Input: part model. Units: mm. Frame: model coordinates. Coordinates: 2 decimals unless noted, no trailing zeros. Loops run counter-clockwise (first coordinate to the right, second up) from the corner with the lowest first, then second, coordinate; pieces in that order, holes last. Notation, with made-up numbers: M 58.25,1.25 L 79.25,1.25 A25 cw 79.25,24.25 Z; hole C 38.5,-36.5 d9. An arc over 180 degrees is marked long. Use a Markdown table: item, result. Add a question column.
1. Section C-C on y = -47. Output: boundary loops of the cut face in (x, z), then the cut area to 3 significant figures.
2. Draft query along X for faces 1 (the flat face through (52, -17, 15)), 2 (the flat face through (54, -35, 15)), 3 (the cylindrical face through (38.49, -40.61, 14.93)). Return one class per face: +X half, -X half, draft (parallel to the pull), parting line (faces both ways), or undercut.
3. Section D-D on x = 19. Output: boundary loops of the cut face in (y, z).
4. Section B-B on z = 14.5. Output: boundary loops of the cut face in (x, y).
5. Section A-A on y = -21. Output: boundary loops of the cut face in (x, z), then the cut area to 3 significant figures.
6. Line query: L1, parallel to X at y = -34, z = 12.75; L2, parallel to X at y = -22, z = 13.25; L3, parallel to Y at x = -23.5, z = 15.5. Output: solid intervals per line, ascending. Write a range as [from, to].
7. Pin query (flat end, axial travel): pin 1 (6 mm diameter, centred on x = -21, z = 11, fed in from +Y); pin 2 (1.8 mm diameter, centred on x = 39.6, y = -39.6, fed in from -Z); pin 3 (2 mm diameter, centred on x = -31, z = 12, fed in from +Y). Return the tip coordinate at first contact, or that it passes through.
```python
from build123d import *

# Parameters (mm, degrees)
CYLINDER875_R               = 1.5
CYLINDER875_DEPTH           = 20
CYLINDER875_PLACEMENT_ANGLE = 45
CYLINDER866_R               = 1.5
CYLINDER866_DEPTH           = 20
CYLINDER869_R               = 1.5
CYLINDER869_DEPTH           = 20
CYLINDER869_PLACEMENT_ANGLE = 135
CYLINDER372_R               = 1.5
CYLINDER372_DEPTH           = 20
CYLINDER377_R               = 1.5
CYLINDER377_DEPTH           = 20
CYLINDER377_PLACEMENT_ANGLE = 225
CYLINDER876_R               = 1.5
CYLINDER876_DEPTH           = 20
CYLINDER873_R               = 1.5
CYLINDER873_DEPTH           = 20
CYLINDER873_PLACEMENT_ANGLE = 45
CYLINDER874_R               = 1.5
CYLINDER874_DEPTH           = 20
CYLINDER867_R               = 52
CYLINDER867_DEPTH           = 10
BOX134_W                    = 108
BOX134_H                    = 36
BOX134_DEPTH                = 10


with BuildPart() as obj1:
    # Cylinder875 → Cylinder875 (new body)
    with BuildSketch(Plane.XY):
        Circle(CYLINDER875_R)
    extrude(amount=CYLINDER875_DEPTH)


with BuildPart() as obj1_1:
    # Cylinder875 placement: moved
    add(obj1.part.moved(Location((39.59798, -39.59798, 2))).rotate(Axis((39.59798, -39.59798, 2), (0, 0, 1)), CYLINDER875_PLACEMENT_ANGLE))


with BuildPart() as obj2:
    # Cylinder866 → Cylinder866 (new body)
    with BuildSketch(Plane(origin=(56, 0, 2), x_dir=(0, 1, 0), z_dir=(0, 0, 1))):
        Circle(CYLINDER866_R)
    extrude(amount=CYLINDER866_DEPTH)


with BuildPart() as obj3:
    # Cylinder869 → Cylinder869 (new body)
    with BuildSketch(Plane.XY):
        Circle(CYLINDER869_R)
    extrude(amount=CYLINDER869_DEPTH)


with BuildPart() as obj3_1:
    # Cylinder869 placement: moved
    add(obj3.part.moved(Location((39.59798, 39.59798, 2))).rotate(Axis((39.59798, 39.59798, 2), (0, 0, 1)), CYLINDER869_PLACEMENT_ANGLE))


with BuildPart() as obj4:
    # Cylinder372 → Cylinder372 (new body)
    with BuildSketch(Plane(origin=(0, 56, 2), x_dir=(-1, 0, 0), z_dir=(0, 0, 1))):
        Circle(CYLINDER372_R)
    extrude(amount=CYLINDER372_DEPTH)


with BuildPart() as obj5:
    # Cylinder377 → Cylinder377 (new body)
    with BuildSketch(Plane.XY):
        Circle(CYLINDER377_R)
    extrude(amount=CYLINDER377_DEPTH)


with BuildPart() as obj5_1:
    # Cylinder377 placement: moved
    add(obj5.part.moved(Location((-39.59798, 39.59798, 2))).rotate(Axis((-39.59798, 39.59798, 2), (0, 0, 1)), CYLINDER377_PLACEMENT_ANGLE))


with BuildPart() as obj6:
    # Cylinder876 → Cylinder876 (new body)
    with BuildSketch(Plane(origin=(-56, 0, 2), x_dir=(0, -1, 0), z_dir=(0, 0, 1))):
        Circle(CYLINDER876_R)
    extrude(amount=CYLINDER876_DEPTH)


with BuildPart() as obj7:
    # Cylinder873 → Cylinder873 (new body)
    with BuildSketch(Plane.XY):
        Circle(CYLINDER873_R)
    extrude(amount=CYLINDER873_DEPTH)


with BuildPart() as obj7_1:
    # Cylinder873 placement: moved
    add(obj7.part.moved(Location((-39.59798, -39.59798, 2))).rotate(Axis((-39.59798, -39.59798, 2), (0, 0, -1)), CYLINDER873_PLACEMENT_ANGLE))


with BuildPart() as compound262:
    # Cylinder874 → Cylinder874 (new body)
    with BuildSketch(Plane(origin=(0, -56, 2), x_dir=(1, 0, 0), z_dir=(0, 0, 1))):
        Circle(CYLINDER874_R)
    extrude(amount=CYLINDER874_DEPTH)

    # Compound262: union obj1, obj2, obj3, obj4, obj5, obj6, obj7
    add(obj1_1.part)
    add(obj2.part)
    add(obj3_1.part)
    add(obj4.part)
    add(obj5_1.part)
    add(obj6.part)
    add(obj7_1.part)


with BuildPart() as obj8:
    # Cylinder867 → Cylinder867 (new body)
    with BuildSketch(Plane.XY.offset(20)):
        Circle(CYLINDER867_R)
    extrude(amount=CYLINDER867_DEPTH)


with BuildPart() as cut151:
    # Box134 → Box134 (new body)
    with BuildSketch(Plane(origin=(-54, -53, 20), x_dir=(1, 0, 0), z_dir=(0, 0, 1))):
        with Locations((54, 18)):
            Rectangle(BOX134_W, BOX134_H)
    extrude(amount=BOX134_DEPTH)

    # Cut152: cut obj8
    add(obj8.part, mode=Mode.SUBTRACT)


with BuildPart() as cut151_1:
    # Cut152 placement: moved
    add(cut151.part.moved(Location((0, 0, -10))))

    # Cut151: cut Compound262
    add(compound262.part, mode=Mode.SUBTRACT)


solid = cut151_1.part
```
Answers below:
| question | item | result |
|---|---|---|
| 1 | outline | M -54,10 L -22.25,10 L -22.25,20 L -54,20 Z; M 22.25,10 L 54,10 L 54,20 L 22.25,20 Z |
| 1 | area | 635 mm² |
| 2 | face 1 | draft |
| 2 | face 2 | +X half |
| 2 | face 3 | undercut |
| 3 | outline | M -53,10 L -48.4,10 L -48.4,20 L -53,20 Z |
| 4 | outline | M -54,-53 L 54,-53 L 54,-17 L 49.14,-17 A52 cw -49.14,-17 L -54,-17 Z; hole C -39.6,-39.6 d3; hole C 39.6,-39.6 d3 |
| 5 | outline | M -54,10 L -47.57,10 L -47.57,20 L -54,20 Z; M 47.57,10 L 54,10 L 54,20 L 47.57,20 Z |
| 5 | area | 129 mm² |
| 6 | L1 | x = [-54, -39.34], [39.34, 54] |
| 6 | L2 | x = [-54, -47.12], [47.12, 54] |
| 6 | L3 | y = [-53, -46.39] |
| 7 | pin 1 | stops at y = -46.13 |
| 7 | pin 2 | passes through |
| 7 | pin 3 | stops at y = -40.99 |
